Can you work these out from the model? Positions are in its coordinate system, mm. Give positions to 0.01 mm unless a question says otherwise; leave off trailing zeros. Write each loop counter-clockwise with the first axis right and the second up, starting at its lowest first coordinate (ties: lowest second). Pieces come first, ordered by that corner, then holes. Notation, with made-up numbers: (59.25, 51) -> (92.25, 51) arc R32 cw to (92.25, 86) -> close; hole circle Ø4 at (68, 10.5). An arc over 180 degrees is marked (long way). Answer as CSV lines item,"result". Start each with the question number.
1. If we section it at C-C on y = 209: Write out the boundary of the cut face in (x, z), plus the area to 3 significant figures.
2. If we section it at D-D on z = 2.25: Count the separate pieces of the cut face and the enclosed holes in it, plus the area to 3 significant figures.
3. I need wall thicknesses on line 1 (Y direction, x = 934, z = 1.3); line 2 (Y direction, x = 760, z = 2.15); line 3 (Y direction, x = 984, z = 3.25). Which ranges of each line are inside material? Lowest first, please. Write a range as [from, to].
4. If we section it at B-B on x = 404: Write out the boundary of the cut face in (y, z), plus the area to 3 significant figures.
5. If we section it at A-A on y = -1: Write out the boundary of the cut face in (x, z), plus the area to 3 significant figures.
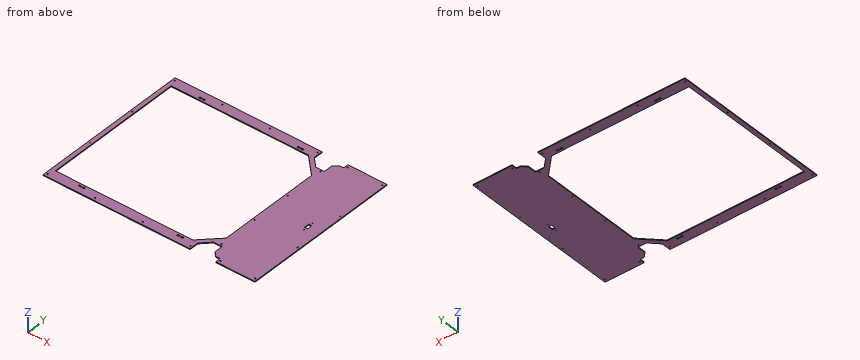
```python
from build123d import *

# Parameters (mm, degrees)
SKETCH_1_W          = 994
SKETCH_1_H          = 748
EXTRUDE_1_DEPTH     = 4
CUT_EXTRUDE_6_DEPTH = 1063.039547286
SKETCH_2_W          = 11.5
SKETCH_2_H          = 6.8
CUT_EXTRUDE_1_DEPTH = 1063.039547286
SKETCH_3_R          = 2.6
CUT_EXTRUDE_4_DEPTH = 1063.039547286
SKETCH_6_R          = 1.75
SKETCH_6_W          = 14
SKETCH_6_H          = 24
CUT_EXTRUDE_7_DEPTH = 1063.039547286
FILLET_1_R          = 2.5


with BuildPart() as part:
    # Эскиз1 → Бобышка-Вытянуть1 (new body)
    with BuildSketch(Plane.XY):
        with Locations((497, 0)):
            Rectangle(SKETCH_1_W, SKETCH_1_H)
        Polygon((20, 327.55), (20, -327.55), (664.165728753, -327.55), (750, -241.715728753), (750, 241.715728753), (664.165728753, 327.55), align=None, mode=Mode.SUBTRACT)
    extrude(amount=EXTRUDE_1_DEPTH)

    # Эскиз5 → Вырез-Вытянуть6 (cut, through all)
    with BuildSketch(Plane.XY.offset(4)):
        Polygon((689.6, 329.834314575), (689.6, 374.4), (810.4, 374.4), (810.4, 349.6), (790.165685425, 349.6), (770.4, 329.834314575), (770.4, 289.6), (729.834314575, 289.6), align=None)
        Polygon((770.4, -329.834314575), (770.4, -289.6), (729.834314575, -289.6), (689.6, -329.834314575), (689.6, -374.4), (810.4, -374.4), (810.4, -349.6), (790.165685425, -349.6), align=None)
    extrude(amount=-CUT_EXTRUDE_6_DEPTH, mode=Mode.SUBTRACT)

    # Эскиз2 → Вырез-Вытянуть1 (cut, through all)
    with BuildSketch(Plane.XY.offset(4)):
        with Locations((607.25, 340.02)):
            Rectangle(SKETCH_2_W, SKETCH_2_H)
        with Locations((624.25, 340.02)):
            Rectangle(SKETCH_2_W, SKETCH_2_H)
        with Locations((624.25, -340.02)):
            Rectangle(SKETCH_2_W, SKETCH_2_H)
        with Locations((607.25, -340.02)):
            Rectangle(SKETCH_2_W, SKETCH_2_H)
        with Locations((145.75, 340.02)):
            Rectangle(SKETCH_2_W, SKETCH_2_H)
        with Locations((162.75, 340.02)):
            Rectangle(SKETCH_2_W, SKETCH_2_H)
        with Locations((145.75, -340.02)):
            Rectangle(SKETCH_2_W, SKETCH_2_H)
        with Locations((162.75, -340.02)):
            Rectangle(SKETCH_2_W, SKETCH_2_H)
    extrude(amount=-CUT_EXTRUDE_1_DEPTH, mode=Mode.SUBTRACT)

    # Эскиз3 → Вырез-Вытянуть4 (cut, through all)
    with BuildSketch(Plane.XY.offset(4)):
        with Locations((10, 360)):
            Circle(SKETCH_3_R)
        with Locations((10, 120)):
            Circle(SKETCH_3_R)
        with Locations((10, -120)):
            Circle(SKETCH_3_R)
        with Locations((10, -360)):
            Circle(SKETCH_3_R)
        with Locations((233.33, 360)):
            Circle(SKETCH_3_R)
        with Locations((456.66, 360)):
            Circle(SKETCH_3_R)
        with Locations((679.99, 360)):
            Circle(SKETCH_3_R)
        with Locations((233.33, -360)):
            Circle(SKETCH_3_R)
        with Locations((456.66, -360)):
            Circle(SKETCH_3_R)
        with Locations((679.99, -360)):
            Circle(SKETCH_3_R)
        with Locations((984, 360)):
            Circle(SKETCH_3_R)
        with Locations((984, 120)):
            Circle(SKETCH_3_R)
        with Locations((984, -120)):
            Circle(SKETCH_3_R)
        with Locations((984, -360)):
            Circle(SKETCH_3_R)
        with Locations((820, -360)):
            Circle(SKETCH_3_R)
        with Locations((820, 360)):
            Circle(SKETCH_3_R)
        with Locations((760, 280)):
            Circle(SKETCH_3_R)
        with Locations((760, 93.33)):
            Circle(SKETCH_3_R)
        with Locations((760, -93.34)):
            Circle(SKETCH_3_R)
        with Locations((760, -280.01)):
            Circle(SKETCH_3_R)
    extrude(amount=-CUT_EXTRUDE_4_DEPTH, mode=Mode.SUBTRACT)

    # Эскиз6 → Вырез-Вытянуть7 (cut, through all)
    with BuildSketch(Plane.XY.offset(4)):
        with Locations((934, 24.8)):
            Circle(SKETCH_6_R)
        with Locations((934, -24.8)):
            Circle(SKETCH_6_R)
        with Locations((934, 0)):
            Rectangle(SKETCH_6_W, SKETCH_6_H)
    extrude(amount=-CUT_EXTRUDE_7_DEPTH, mode=Mode.SUBTRACT)

    # Скругление1
    fillet_1_edges = [part.edges().sort_by_distance(p)[0] for p in [
        (689.6, 329.834314575, 2),
        (729.834314575, 289.6, 2),
        (810.4, 349.6, 2),
        (790.165685425, 349.6, 2),
        (770.4, 329.834314575, 2),
        (770.4, 289.6, 2),
        (810.4, -349.6, 2),
        (689.6, -329.834314575, 2),
        (729.834314575, -289.6, 2),
        (770.4, -289.6, 2),
        (770.4, -329.834314575, 2),
        (790.165685425, -349.6, 2),
    ]]
    fillet(fillet_1_edges, radius=FILLET_1_R)


solid = part.part
```
Computed values:
1,outline,"(0, 0) -> (20, 0) -> (20, 4) -> (0, 4) -> close; (750, 0) -> (994, 0) -> (994, 4) -> (750, 4) -> close"
1,area,"1,060 mm2"
2,separate pieces,"1"
2,enclosed holes,"32"
2,area,"257,000 mm2"
3,line 1,"y = [-374, -26.55], [-23.05, -12], [12, 23.05], [26.55, 374]"
3,line 2,"y = [-289.6, -282.61], [-277.41, -95.94], [-90.74, 90.73], [95.93, 277.4], [282.6, 289.6]"
3,line 3,"y = [-374, -362.6], [-357.4, -122.6], [-117.4, 117.4], [122.6, 357.4], [362.6, 374]"
4,outline,"(-374, 0) -> (-327.55, 0) -> (-327.55, 4) -> (-374, 4) -> close; (327.55, 0) -> (374, 0) -> (374, 4) -> (327.55, 4) -> close"
4,area,"372 mm2"
5,outline,"(0, 0) -> (20, 0) -> (20, 4) -> (0, 4) -> close; (750, 0) -> (927, 0) -> (927, 4) -> (750, 4) -> close; (941, 0) -> (994, 0) -> (994, 4) -> (941, 4) -> close"
5,area,"1,000 mm2"
